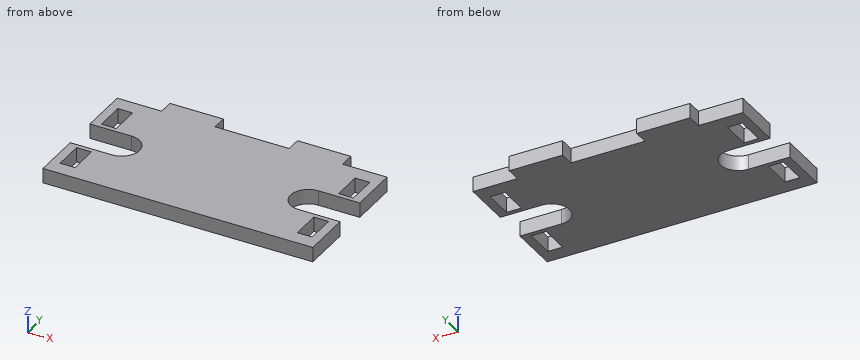
from build123d import *

# Parameters (mm, degrees)
F0_W     = 5
F0_H     = 10
F1_DEPTH = 5


with BuildPart() as f1:
    # F0 (on Top) → F1 (new body)
    with BuildSketch(Plane.XY):
        with BuildLine():
            Line((-30.5, 22.5), (-45.5, 22.5))
            Line((-45.5, 22.5), (-45.5, 6))
            Line((-45.5, 6), (-31.5, 6))
            ThreePointArc((-31.5, 6), (-25.5, 0), (-31.5, -6))
            Line((-31.5, -6), (-45.5, -6))
            Line((-45.5, -6), (-45.5, -22.5))
            Line((-45.5, -22.5), (45.5, -22.5))
            Line((45.5, -22.5), (45.5, -6))
            Line((45.5, -6), (31.5, -6))
            ThreePointArc((31.5, -6), (25.5, 0), (31.5, 6))
            Line((31.5, 6), (45.5, 6))
            Line((45.5, 6), (45.5, 22.5))
            Line((45.5, 22.5), (30.5, 22.5))
            Line((30.5, 22.5), (30.5, 27.5))
            Line((30.5, 27.5), (12.5, 27.5))
            Line((12.5, 27.5), (12.5, 22.5))
            Line((12.5, 22.5), (-12.5, 22.5))
            Line((-12.5, 22.5), (-12.5, 27.5))
            Line((-12.5, 27.5), (-30.5, 27.5))
            Line((-30.5, 27.5), (-30.5, 22.5))
        make_face()
        with Locations((-40, -12.5)):
            Rectangle(F0_W, F0_H, mode=Mode.SUBTRACT)
        with Locations((40, -12.5)):
            Rectangle(F0_W, F0_H, mode=Mode.SUBTRACT)
        with Locations((-40, 12.5)):
            Rectangle(F0_W, F0_H, mode=Mode.SUBTRACT)
        with Locations((40, 12.5)):
            Rectangle(F0_W, F0_H, mode=Mode.SUBTRACT)
    extrude(amount=F1_DEPTH)


solid = f1.part
The listing builds one solid part. Answer for the finished solid, in the listing's coordinates (mm). Give positions to 0.01 mm unless a question says otherwise; leave off trailing zeros. Write each loop counter-clockwise with the first axis right and the second up, starting at its lowest first coordinate (ties: lowest second). Pieces come first, ordered by that corner, then holes. Notation, with made-up numbers: (-34, 25) -> (4, 25) arc R10 cw to (4, 29) -> close; hole circle Ø7 at (70, -8.5). An arc over 180 degrees is marked (long way). Use a Markdown table: item, result.
(1) Find the intervals of material crossed by probe 1 along X at (y, z) = (16.5, 3.8); probe 2 along Y at (x, z) = (42, 3.6); probe 3 along X at (y, z) = (24.5, 0.3), in increasing order. Write a range as from..to.
Return value:
| item | result |
|---|---|
| probe 1 | -45.5..-42.5, -37.5..37.5, 42.5..45.5 |
| probe 2 | -22.5..-17.5, -7.5..-6, 6..7.5, 17.5..22.5 |
| probe 3 | -30.5..-12.5, 12.5..30.5 |
(2) Section D-D, the plane z = 3.4 is taken. Give the number of separate pieces and of enclosed holes in the cut face, then the cut area to 3 significant figures.
Return value:
| item | result |
|---|---|
| separate pieces | 1 |
| enclosed holes | 4 |
| area | 3,630 mm2 |
(3) Section C-C, the plane x = -4.5 is taken. Determine the outline of the cut face in (y, z).
Return value:
| item | result |
|---|---|
| outline | (-22.5, 0) -> (22.5, 0) -> (22.5, 5) -> (-22.5, 5) -> close |
(4) Section A-A, the plane y = 13.5 is taken. Determine the outline of the cut face in (x, z), then the cut area to 3 significant figures.
Return value:
| item | result |
|---|---|
| outline | (-45.5, 0) -> (-42.5, 0) -> (-42.5, 5) -> (-45.5, 5) -> close; (-37.5, 0) -> (37.5, 0) -> (37.5, 5) -> (-37.5, 5) -> close; (42.5, 0) -> (45.5, 0) -> (45.5, 5) -> (42.5, 5) -> close |
| area | 405 mm2 |
(5) Section B-B, the plane x = 33.5 is taken. Determine the outline of the cut face in (y, z).
Return value:
| item | result |
|---|---|
| outline | (-22.5, 0) -> (-6, 0) -> (-6, 5) -> (-22.5, 5) -> close; (6, 0) -> (22.5, 0) -> (22.5, 5) -> (6, 5) -> close |
(6) Flat-ended cylindrical pins translate along their axes: P1, Ø2.5, axis at x = 41, z = 3.5, coming from the +Y side; P2, Ø2.5, axis at y = 25, z = 2.5, coming from the +X side. Find the tip coordinate at first contact, or state that the pin passes through.
Return value:
| item | result |
|---|---|
| P1 | y = 22.5 |
| P2 | x = 30.5 |
